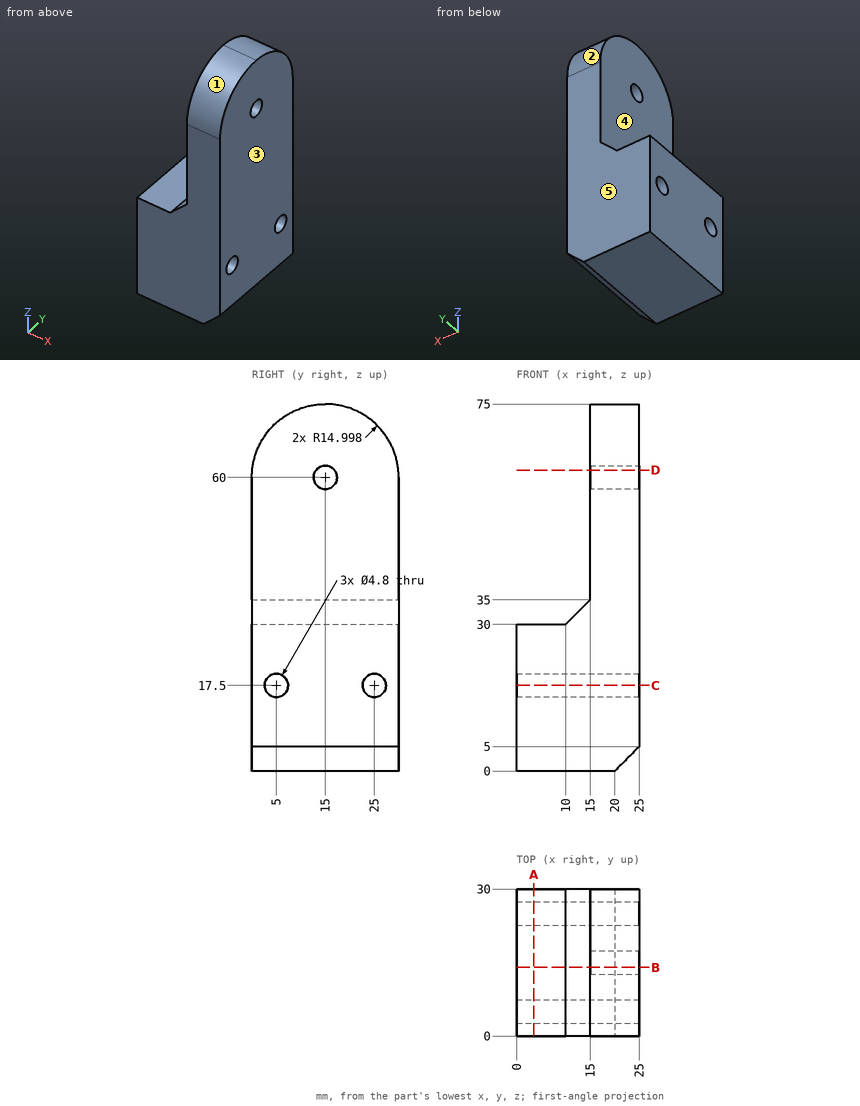
The drawing under review shows one solid part. Ordinate dimensions are in mm from its lowest x, y, z. A direction names the side the tool comes from. Give positions to 0.01 mm unless a question says otherwise; leave off trailing zeros. Write each loop counter-clockwise with the first axis right and the second up, starting at its lowest first coordinate (ties: lowest second). Pieces come first, ordered by that corner, then holes. Notation, with made-up numbers: (36, 10.5) -> (46, 10.5) arc R14 ccw to (46, 37.5) -> close; hole circle Ø6 at (43.25, -28.75). An arc over 180 degrees is marked (long way). Put each result on its own line as item: value.
(1) To check wall thickness, follow probe 1 along Y at (x, z) = (6.5, 17.5); probe 2 along Y at (x, z) = (20.75, 60); probe 3 along Y at (x, z) = (1.75, 18). State the ranges of each line that lie inside material, in increasing order. Write a range as from..to.
Results are:
probe 1: 0..2.6, 7.4..22.6, 27.4..30
probe 2: 0..12.6, 17.4..30
probe 3: 0..2.65, 7.35..22.65, 27.35..30
(2) We need section C-C, the plane z = 17.5. Give the boundary of the cut face in (x, y).
Results are:
outline: (0, 0) -> (25, 0) -> (25, 2.6) -> (0, 2.6) -> close; (0, 7.4) -> (25, 7.4) -> (25, 22.6) -> (0, 22.6) -> close; (0, 27.4) -> (25, 27.4) -> (25, 30) -> (0, 30) -> close
(3) The part is to be moulded in two halves that separate along Y. For the marked faces 1, 2 and 3, say which applies: pulls with the +Y half, pulls with the -Y half, needs draft (parallel to the pull), parting line crosses it, or undercut.
Results are:
face 1: pulls with the -Y half
face 2: pulls with the +Y half
face 3: needs draft
(4) We need section B-B, the plane y = 14. Give the boundary of the cut face in (x, z).
Results are:
outline: (0, 0) -> (20, 0) -> (25, 5) -> (25, 57.82) -> (15, 57.82) -> (15, 35) -> (10, 30) -> (0, 30) -> close; (15, 62.18) -> (25, 62.18) -> (25, 74.97) -> (15, 74.97) -> close
(5) We need section D-D, the plane z = 61.5. Give the boundary of the cut face in (x, y) (1 decimal), and give its area (3 significant figures).
Results are:
outline: (15, 0.1) -> (25, 0.1) -> (25, 13.1) -> (15, 13.1) -> close; (15, 16.9) -> (25, 16.9) -> (25, 29.9) -> (15, 29.9) -> close
area: 261 mm²
(6) For pin 1 Ø3 at (x, y) = (3, 16) entering from +Z; pin 2 Ø4 at (x, y) = (18, 5.5) entering from +Z; pin 3 Ø5.5 at (y, z) = (15, 60) entering from -X, all flat-tipped, find the tip position at first contact; note any pin that passes through.
Results are:
pin 1: z = 30
pin 2: z = 72.99
pin 3: x = 15
(7) Tool access review of the marked faces 4 and 5: name each direction out of +Z, -Z, +X, -X, +Y, -Y from which nothing blocks a thin tool from reaching the whole face with its end or side.
Results are:
face 4: +Z, -X, +Y, -Y
face 5: +Z, -Z, +X, -X, +Y
(8) We need section A-A, the plane x = 3.5. Give the boundary of the cut face in (y, z).
Results are:
outline: (0, 0) -> (30, 0) -> (30, 30) -> (0, 30) -> close; hole circle Ø4.8 at (5, 17.5); hole circle Ø4.8 at (25, 17.5)
